The model under review builds one solid part; all positions refer to its coordinate system, in mm. A direction names the side the tool comes from. Give positions to 0.01 mm unless a question says otherwise; leave off trailing zeros. Order: outer loops, then holes, each group sorted by start corner. A loop starts at its lowest first (then second) coordinate and runs counter-clockwise, first axis right, second up. Notation, with made-up numbers: (89.5, 8) - (126.5, 8) arc R23 ccw to (126.5, 19) - close; hole circle Ø4 at (57, -11.5). An arc over 180 degrees is marked (long way). Put each result on its own line as item: value.
```python
from build123d import *

# Parameters (mm, degrees)
SKETCH_1_W      = 19
SKETCH_1_H      = 52
SKETCH_1_W_2    = 60
SKETCH_1_H_2    = 60
SKETCH_1_H_3    = 106.4
SKETCH_1_H_4    = 111
SKETCH_1_H_5    = 111.3
SKETCH_1_H_6    = 112
SKETCH_1_H_7    = 113
SKETCH_1_H_8    = 116.5
SKETCH_1_H_9    = 131.6
EXTRUDE_1_DEPTH = 1
EXTRUDE_2_DEPTH = 1
EXTRUDE_3_DEPTH = 33.212704
SKETCH_4_W      = 0.5
SKETCH_4_H      = 27
EXTRUDE_4_DEPTH = 42
SKETCH_5_W      = 0.5
SKETCH_5_H      = 27
EXTRUDE_5_DEPTH = 18
EXTRUDE_6_DEPTH = 1
EXTRUDE_7_DEPTH = 15


with BuildPart() as part:
    # 草图1 → 拉伸1 (new body)
    with BuildSketch(Plane.XY):
        with Locations((858.7, -476.2)):
            Rectangle(SKETCH_1_W, SKETCH_1_H)
        Polygon((825.5, -1174.6), (825.5, -1125.1), (765.5, -1125.1), (761.5, -1125.1), (761.5, -1174.6), (765.5, -1174.6), align=None)
        Polygon((849.2, -1121.1), (909.2, -1121.1), (909.2, -1091.6), (909.2, -1064), (849.2, -1064), align=None)
        with Locations((795.5, -474.2)):
            Rectangle(SKETCH_1_W_2, SKETCH_1_H_2)
        with Locations((879.2, -559.9)):
            Rectangle(SKETCH_1_W_2, SKETCH_1_H_3)
        Polygon((909.2, -953.1), (849.2, -953.1), (849.2, -1050.1), (849.2, -1064), (909.2, -1064), align=None)
        with Locations((795.5, -953.1)):
            Rectangle(SKETCH_1_W_2, SKETCH_1_H_4)
        with Locations((795.5, -842.1)):
            Rectangle(SKETCH_1_W_2, SKETCH_1_H_4)
        with Locations((879.2, -897.45)):
            Rectangle(SKETCH_1_W_2, SKETCH_1_H_5)
        with Locations((795.5, -560.2)):
            Rectangle(SKETCH_1_W_2, SKETCH_1_H_6)
        with Locations((795.5, -730.1)):
            Rectangle(SKETCH_1_W_2, SKETCH_1_H_7)
        with Locations((795.5, -1066.85)):
            Rectangle(SKETCH_1_W_2, SKETCH_1_H_8)
        with Locations((879.2, -776)):
            Rectangle(SKETCH_1_W_2, SKETCH_1_H_9)
        Polygon((849.2, -1121.1), (909.2, -1121.1), (1031.2, -1121.1), (1031.2, -1174.6), (849.2, -1174.6), align=None)
        with BuildLine():
            Line((1213.4, -757.7), (1226.4, -727))
            ThreePointArc((1226.4, -727), (1075.34720829, -664.295577574), (916.2, -626.6))
            Line((916.2, -626.6), (916.2, -623.1))
            Line((916.2, -623.1), (849.2, -623.1))
            Line((849.2, -623.1), (849.2, -668.1))
            Line((849.2, -668.1), (849.2, -681.1))
            Line((849.2, -681.1), (849.2, -710.2))
            Line((849.2, -710.2), (909.2, -710.2))
            Line((909.2, -710.2), (909.2, -668.1))
            Line((909.2, -668.1), (916.2, -668.1))
            Line((916.2, -668.1), (916.2, -664.6))
            ThreePointArc((916.2, -664.6), (1067.153405165, -703.637303814), (1213.4, -757.7))
        make_face()
        Polygon((765.5, -616.2), (825.5, -616.2), (825.5, -504.2), (825.5, -444.2), (849.2, -444.2), (849.2, -450.2), (849.2, -502.2), (849.2, -506.7), (849.2, -613.1), (849.2, -623.1), (849.2, -668.1), (849.2, -681.1), (849.2, -710.2), (849.2, -841.8), (849.2, -953.1), (849.2, -1050.1), (849.2, -1064), (849.2, -1121.1), (849.2, -1174.6), (825.5, -1174.6), (825.5, -1125.1), (825.5, -1008.6), (825.5, -897.6), (825.5, -786.6), (825.5, -673.6), (765.5, -673.6), (727.5, -673.6), (727.5, -616.2), align=None)
    extrude(amount=-EXTRUDE_1_DEPTH)

    # 草图2 → 拉伸2 (add)
    with BuildSketch(Plane.XY):
        Polygon((1237.099840045, -739.006390924), (1239.746814184, -733.845622773), (1226.4, -727), (1213.4, -757.7), (1226.746814184, -764.545622773), (1224.14778512, -769.612913087), (1235.545483088, -774.927746934), (1249.581778451, -744.826814391), align=None)
    extrude(amount=-EXTRUDE_2_DEPTH)

    # 草图3 → 拉伸3 (add)
    with BuildSketch(Plane(origin=(-76.138469502, -163.279474765, 0), x_dir=(0.9063077870373919, -0.42261826173910827, 0), z_dir=(-0.42261826173910827, -0.9063077870373919, 0))):
        Polygon((1447.283109945, 0), (1477.783109945, 15), (1477.783109945, 14.5), (1447.283109945, -0.5), align=None)
    extrude(amount=-EXTRUDE_3_DEPTH)

    # 草图4 → 拉伸4 (add)
    with BuildSketch(Plane(origin=(999.7, -1174.6, 0), x_dir=(0, 0, -1), z_dir=(1, 0, 0))):
        with Locations((-20.608674231, 109)):
            Rectangle(SKETCH_4_W, SKETCH_4_H)
        Polygon((-20.858674231, 95.5), (0, 53.5), (0.5, 53.5), (-20.358674231, 95.5), align=None)
    extrude(amount=-EXTRUDE_4_DEPTH)

    # 草图5 → 拉伸5 (add)
    with BuildSketch(Plane(origin=(999.7, -1174.6, 0), x_dir=(0, 0, -1), z_dir=(1, 0, 0))):
        with Locations((-20.608674231, 109)):
            Rectangle(SKETCH_5_W, SKETCH_5_H)
        Polygon((-41.858674231, 53.5), (-41.358674231, 53.5), (-20.358674231, 95.5), (-20.858674231, 95.5), align=None)
    extrude_5 = extrude(amount=EXTRUDE_5_DEPTH)

    # 镜像1: 拉伸5 across plane
    add(extrude_5.mirror(Plane(origin=(978.7, -1174.6, 0), x_dir=(0, 0, 1), z_dir=(-1, 0, 0))))

    # 草图6 → 拉伸6 (add)
    with BuildSketch(Plane.XY):
        Polygon((1031.2, -1121.1), (1117.8, -1121.1), (1091.336296883, -1177.851594476), (1068.2, -1174.6), (1031.2, -1174.6), align=None)
    extrude(amount=-EXTRUDE_6_DEPTH)

    # 草图7 → 拉伸7 (add)
    with BuildSketch(Plane(origin=(1109.136325634, -1139.679309634, 0), x_dir=(0.9063077870366769, -0.422618261740642, 0), z_dir=(-0.422618261740642, -0.9063077870366769, 0))):
        Polygon((-30, -0.5), (0, 14.5), (0, 15), (-30, 0), align=None)
    extrude(amount=EXTRUDE_7_DEPTH)


solid = part.part
```
(1) Clearance check with flat-ended pins moving along their axes: pin 1 Ø0.8 at (x, z) = (888, -0.5) entering from +Y; pin 2 Ø1.1 at (x, z) = (746, -0.5) entering from -Y; pin 3 Ø0.8 at (y, z) = (-476.5, -0.5) entering from +X; pin 4 Ø12 at (x, z) = (1170, 11) entering from +Y. State where each tip first meets the part, or that it passes through.
The answers:
pin 1: y = -506.7
pin 2: y = -673.6
pin 3: x = 868.2
pin 4: through
(2) For faces 4 (the flat face through (1242.465, -760.088, -0.826)), 5 (the flat face through (1017.7, -1084, 23)), list the 3-axis set-ups (+Z, -Z, +X, -X, +Y, -Y) from which the entire face can be reached by the end or side of a thin tool; tool diameter is ignored.
The answers:
face 4: -Z, +X, -Y
face 5: +Z, -Z, +X, +Y, -Y
(3) The part is to be moulded in two halves that separate along X. For faces 1 (the flat face through (1104.753, -1149.079, -0.493)), 2 (the cylindrical face through (1065.069, -702.986, -0.493)), 3 (the flat face through (979, -1066, 20.359)), say which applies: pulls with the +X half, pulls with the -X half, needs draft (parallel to the pull), parting line crosses it, or undercut.
The answers:
face 1: pulls with the +X half
face 2: undercut
face 3: needs draft
(4) Take a section at D-D, the plane x = 1173. Write out the cut boundary in (y, z), then the cut area to 3 significant figures.
The answers:
outline: (-741.07, -1) - (-701.54, -1) - (-701.54, 0) - (-741.07, 0) - close
area: 39.5 mm^2
(5) Take a section at C-C, the plane y = -874.5. Write out the cut boundary in (x, z), then the cut area to 3 significant figures.
The answers:
outline: (765.5, -1) - (909.2, -1) - (909.2, 0) - (765.5, 0) - close
area: 144 mm^2
(6) Take a section at A-A, the plane z = 34.5. Write out the cut boundary in (x, y), then the cut area to 3 significant figures.
The answers:
outline: (939.7, -1107.38) - (957.7, -1107.38) - (957.7, -1106.38) - (939.7, -1106.38) - close; (999.7, -1107.38) - (1017.7, -1107.38) - (1017.7, -1106.38) - (999.7, -1106.38) - close
area: 36.0 mm^2
(7) Take a section at B-B, the plane x = 928. Write out the cut boundary in (y, z), then the cut area to 3 significant figures.
The answers:
outline: (-1174.6, -1) - (-1121.1, -1) - (-1121.1, 0) - (-1174.6, 0) - close; (-667.07, -1) - (-628.48, -1) - (-628.48, 0) - (-667.07, 0) - close
area: 92.1 mm^2
(8) Wall thickness on L1, parallel to Z at x = 787, y = -886.5; L2, parallel to Y at x = 996, z = 16: over which ranges is each line inside the solid? List them lowest first.
The answers:
L1: -1 to 0
L2: -1088.88 to -1087.88
